Verification items for this drawing (mm, ordinates from the low corner). A direction names the side the tool comes from. Round coordinates to 2 decimals unless told otherwise and drop trailing zeros. Loops run counter-clockwise (first coordinate to the right, second up) from the corner with the lowest first, then second, coordinate; pieces in that order, holes last. Notation, with made-up numbers: (8, 48) - (26, 48) arc R21 ccw to (26, 82) - close; hole circle Ø5 at (2, 47.25). An arc over 180 degrees is marked (long way). Answer in a Markdown table with one row per item. Add a question column.
(1) Mould release check, pull along Z, two halves, no side actions. Record for the marked faces 3, 4 and 5: +Z half, -Z half, draft (parallel to the pull), parting line (faces both ways), or undercut.
(2) Access from +Z, -Z, +X, -X, +Y, -Y to the whole of each face (thin tool, end or side, straight path). Record for the marked faces 1 and 2.
(3) Gauge pin test, flat ends, axial feed: pin 1 (1.5 mm diameter, centred on y = 6, z = 3, fed in from -X); pin 2 (4 mm diameter, centred on y = 5.5, z = 12.5, fed in from +X). Record the tip position at first contact, or that the pin passes through.
(4) Cross-section at C-C on z = 18. Enter the section's corners in (x, y).
(5) Cross-section at D-D on y = 1. Enter the section's corners in (x, z).
(6) Thickness scan on line 1 along X through (y, z) = (3.25, 11); line 2 along Y through (x, z) = (6, 2.75); line 3 along Z through (x, y) = (10.75, 0.75). Record the ranges inside material, lowest first.
(7) Cross-section at A-A on x = 11. Enter the section's corners in (y, z), then the cut area to 3 significant figures.
(8) Cross-section at B-B on z = 11. Enter the section's corners in (x, y), then the cut area to 3 significant figures.
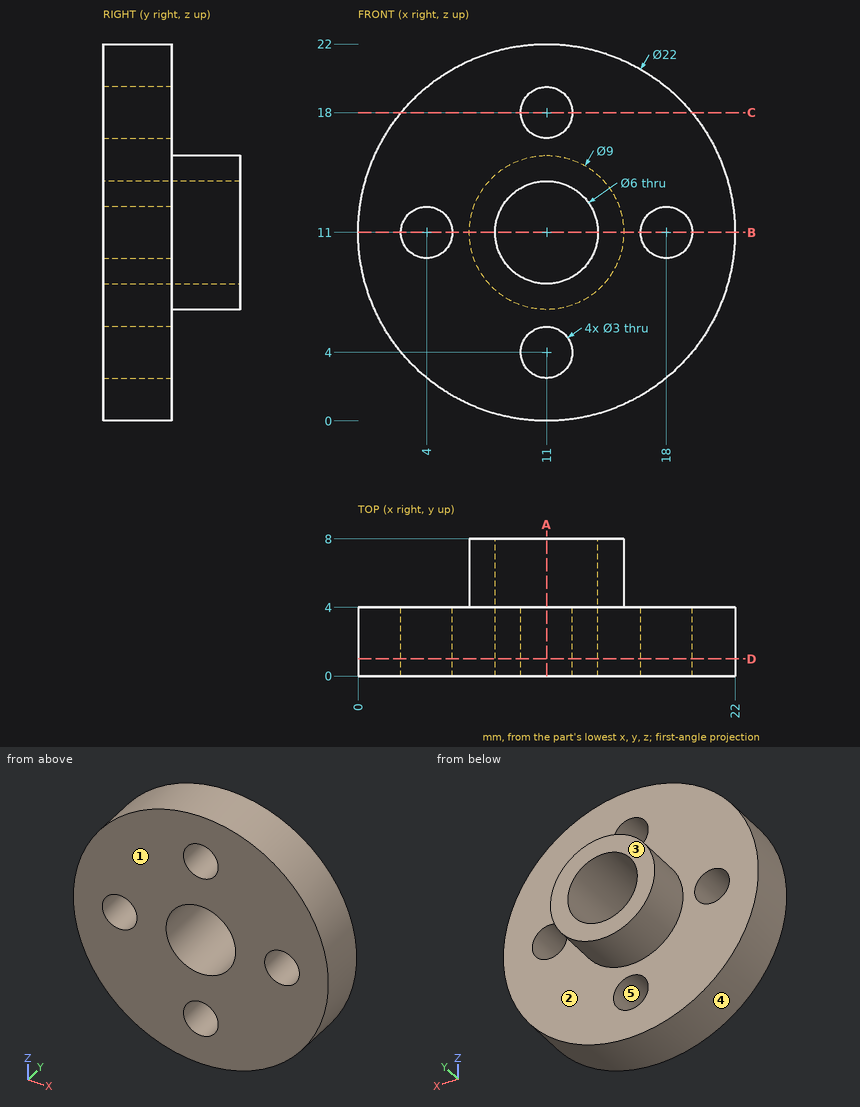
Answers:
| question | item | result |
|---|---|---|
| 1 | face 3 | draft |
| 1 | face 4 | parting line |
| 1 | face 5 | undercut |
| 2 | face 1 | +Z, -Z, +X, -X, -Y |
| 2 | face 2 | +Y |
| 3 | pin 1 | passes through |
| 3 | pin 2 | stops at x = 22 |
| 4 | outline | (2.51, 0) - (9.5, 0) - (9.5, 4) - (2.51, 4) - close; (12.5, 0) - (19.49, 0) - (19.49, 4) - (12.5, 4) - close |
| 5 | outline | circle Ø22 at (11, 11); hole circle Ø3 at (4, 11); hole circle Ø6 at (11, 11); hole circle Ø3 at (11, 4); hole circle Ø3 at (11, 18); hole circle Ø3 at (18, 11) |
| 6 | line 1 | x = 0 to 2.5, 5.5 to 8, 14 to 16.5, 19.5 to 22 |
| 6 | line 2 | y = 0 to 4 |
| 6 | line 3 | z = 0 to 2.52, 5.48 to 8.01, 13.99 to 16.52, 19.48 to 22 |
| 7 | outline | (0, 0) - (4, 0) - (4, 2.5) - (0, 2.5) - close; (0, 5.5) - (4, 5.5) - (4, 6.5) - (8, 6.5) - (8, 8) - (0, 8) - close; (0, 14) - (8, 14) - (8, 15.5) - (4, 15.5) - (4, 16.5) - (0, 16.5) - close; (0, 19.5) - (4, 19.5) - (4, 22) - (0, 22) - close |
| 7 | area | 52.0 mm^2 |
| 8 | outline | (0, 0) - (2.5, 0) - (2.5, 4) - (0, 4) - close; (5.5, 0) - (8, 0) - (8, 8) - (6.5, 8) - (6.5, 4) - (5.5, 4) - close; (14, 0) - (16.5, 0) - (16.5, 4) - (15.5, 4) - (15.5, 8) - (14, 8) - close; (19.5, 0) - (22, 0) - (22, 4) - (19.5, 4) - close |
| 8 | area | 52.0 mm^2 |
